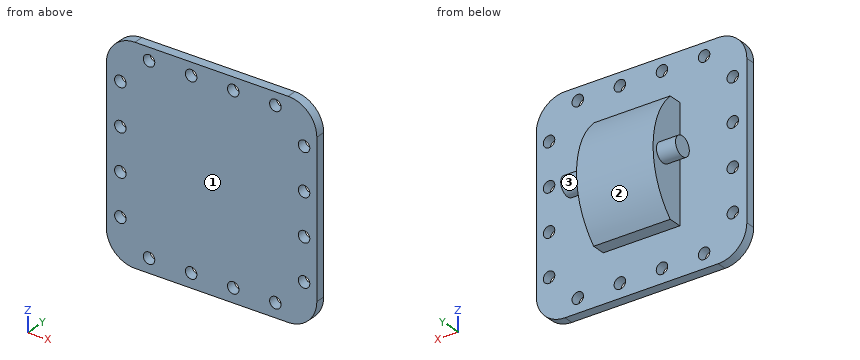
from build123d import *

# Parameters (mm, degrees)
SKETCH1_W                = 110
SKETCH1_H                = 110
BOSS_EXTRUDE1_DEPTH      = 5
FILLET2_R                = 15
FILLET3_R                = 15
FILLET4_R                = 15
FILLET5_R                = 15
SKETCH2_W                = 40
SKETCH2_H                = 60
BOSS_EXTRUDE2_DEPTH      = 24
BOSS_EXTRUDE3_DEPTH      = 10
BOSS_EXTRUDE3_DEPTH_BACK = 50
SKETCH4_R                = 5
FILLET6_R                = 10
FILLET7_R                = 10
SKETCH5_R                = 3
CUT_EXTRUDE1_DEPTH       = 10
CUT_EXTRUDE2_DEPTH       = 60


with BuildPart() as part:
    # Sketch1 → Boss-Extrude1 (new body)
    with BuildSketch(Plane(origin=(0, 0, 0), x_dir=(1, 0, 0), z_dir=(0, 1, 0))):
        Rectangle(SKETCH1_W, SKETCH1_H)
    extrude(amount=BOSS_EXTRUDE1_DEPTH)

    # Fillet2
    fillet2_edges = [part.edges().sort_by_distance(p)[0] for p in [
        (55, 2.5, -55),
    ]]
    fillet(fillet2_edges, radius=FILLET2_R)

    # Fillet3
    fillet3_edges = [part.edges().sort_by_distance(p)[0] for p in [
        (-55, 2.5, -55),
    ]]
    fillet(fillet3_edges, radius=FILLET3_R)

    # Fillet4
    fillet4_edges = [part.edges().sort_by_distance(p)[0] for p in [
        (-55, 2.5, 55),
    ]]
    fillet(fillet4_edges, radius=FILLET4_R)

    # Fillet5
    fillet5_edges = [part.edges().sort_by_distance(p)[0] for p in [
        (55, 2.5, 55),
    ]]
    fillet(fillet5_edges, radius=FILLET5_R)

    # Sketch2 → Boss-Extrude2 (add)
    with BuildSketch(Plane(origin=(0, 5, 0), x_dir=(1, 0, 0), z_dir=(0, 1, 0))):
        Rectangle(SKETCH2_W, SKETCH2_H)
    extrude(amount=BOSS_EXTRUDE2_DEPTH)

    # Sketch4 → Boss-Extrude3 (add, two sides: drawn at the far end of the back side and taken through both)
    with BuildSketch(Plane(origin=(20, 0, 0), x_dir=(0, 0, -1), z_dir=(1, 0, 0)).offset(-BOSS_EXTRUDE3_DEPTH_BACK)):
        with Locations((0, 17)):
            Circle(SKETCH4_R)
    extrude(amount=BOSS_EXTRUDE3_DEPTH + BOSS_EXTRUDE3_DEPTH_BACK)

    # Fillet6
    fillet6_edges = [part.edges().sort_by_distance(p)[0] for p in [
        (0, 29, 30),
    ]]
    fillet(fillet6_edges, radius=FILLET6_R)

    # Fillet7
    fillet7_edges = [part.edges().sort_by_distance(p)[0] for p in [
        (0, 29, -30),
    ]]
    fillet(fillet7_edges, radius=FILLET7_R)

    # Sketch5 → Cut-Extrude1 (cut)
    with BuildSketch(Plane.XZ):
        with Locations(Location((48.334696306, -10.581629618, 0), (0, 0, 270))):
            Circle(SKETCH5_R)
        with Locations(Location((48.334696306, 33.418370382, 0), (0, 0, 270))):
            Circle(SKETCH5_R)
        with Locations(Location((-47.665303694, 11.418370382, 0), (0, 0, 270))):
            Circle(SKETCH5_R)
        with Locations(Location((-47.665303694, -10.581629618, 0), (0, 0, 270))):
            Circle(SKETCH5_R)
        with Locations(Location((-47.665303694, -32.581629618, 0), (0, 0, 270))):
            Circle(SKETCH5_R)
        with Locations(Location((-32.665303694, -47.581629618, 0), (0, 0, 270))):
            Circle(SKETCH5_R)
        with Locations(Location((-10.665303694, -47.581629618, 0), (0, 0, 270))):
            Circle(SKETCH5_R)
        with Locations(Location((11.334696306, -47.581629618, 0), (0, 0, 270))):
            Circle(SKETCH5_R)
        with Locations(Location((33.334696306, -47.581629618, 0), (0, 0, 270))):
            Circle(SKETCH5_R)
        with Locations(Location((48.334696306, -32.581629618, 0), (0, 0, 270))):
            Circle(SKETCH5_R)
        with Locations(Location((48.334696306, 11.418370382, 0), (0, 0, 270))):
            Circle(SKETCH5_R)
        with Locations(Location((33.334696306, 48.418370382, 0), (0, 0, 270))):
            Circle(SKETCH5_R)
        with Locations(Location((11.334696306, 48.418370382, 0), (0, 0, 270))):
            Circle(SKETCH5_R)
        with Locations(Location((-10.665303694, 48.418370382, 0), (0, 0, 270))):
            Circle(SKETCH5_R)
        with Locations(Location((-32.665303694, 48.418370382, 0), (0, 0, 270))):
            Circle(SKETCH5_R)
        with Locations(Location((-47.665303694, 33.418370382, 0), (0, 0, 270))):
            Circle(SKETCH5_R)
    extrude(amount=-CUT_EXTRUDE1_DEPTH, mode=Mode.SUBTRACT)

    # Sketch6 → Cut-Extrude2 (cut)
    with BuildSketch(Plane(origin=(20, 0, 0), x_dir=(0, 0, -1), z_dir=(1, 0, 0))):
        with BuildLine():
            Line((30, 19), (30, 12))
            ThreePointArc((30, 12), (0, 24.426406871), (-30, 12))
            Line((-30, 12), (-30, 19))
            ThreePointArc((-30, 19), (-27.071067812, 26.071067812), (-20, 29))
            Line((-20, 29), (20, 29))
            ThreePointArc((20, 29), (27.071067812, 26.071067812), (30, 19))
        make_face()
    extrude(amount=-CUT_EXTRUDE2_DEPTH, mode=Mode.SUBTRACT)


solid = part.part
Check sheet for the modelled part. Datum: model origin and axes. Units: mm. Face numbers are marked on the shaded views. Round coordinates to 2 decimals unless told otherwise and drop trailing zeros. Loops run counter-clockwise (first coordinate to the right, second up) from the corner with the lowest first, then second, coordinate; pieces in that order, holes last. Notation, with made-up numbers: (60.25, 4) -> (104.25, 4) arc R23 ccw to (104.25, 37) -> close; hole circle Ø1 at (51, 17.5). An arc over 180 degrees is marked (long way). Put each result on its own line as item: value. Start each with the question number.
1. Section check B-B (z = 0). Enter the section's corners in (x, y), plus the area to 3 significant figures.
2. Gauge pin test, flat ends, axial feed: pin 1 (7 mm diameter, centred on x = 11.33, z = -47.58, fed in from +Y); pin 2 (5.5 mm diameter, centred on x = 9, y = 9, fed in from +Z); pin 3 (5.5 mm diameter, centred on x = -10.67, z = 48.42, fed in from -Y); pin 4 (12 mm diameter, centred on y = 11.5, z = 21.5, fed in from -X). Record the tip position at first contact, or that the pin passes through.
3. Section check C-C (y = 19). Enter the section's corners in (x, z), plus the area to 3 significant figures.
4. Section check D-D (z = 18.5). Enter the section's corners in (x, y).
5. Scan lines: probe 1 along X at (y, z) = (4, 12.5); probe 2 along Y at (x, z) = (-39, 18.5); probe 3 along Z at (x, y) = (0.5, 6). Record each from-to range of solid material in increasing order.
6. Section check A-A (x = -27.5). Enter the section's corners in (y, z), plus the area to 3 significant figures.
7. Draft check along Y on the marked faces 1, 2 and 3. Enter one of: +Y half, -Y half, draft (parallel to the pull), parting line (faces both ways), or undercut.
Findings:
1. outline: (-55, 0) -> (55, 0) -> (55, 5) -> (20, 5) -> (20, 12) -> (30, 12) -> (30, 22) -> (20, 22) -> (20, 24.43) -> (-20, 24.43) -> (-20, 22) -> (-30, 22) -> (-30, 12) -> (-20, 12) -> (-20, 5) -> (-55, 5) -> close
1. area: 1,530 mm^2
2. pin 1: stops at y = 5
2. pin 2: stops at z = 30
2. pin 3: passes through
2. pin 4: stops at x = -20
3. outline: (-30, -4.58) -> (-20, -4.58) -> (-20, -20.76) -> (20, -20.76) -> (20, -4.58) -> (30, -4.58) -> (30, 4.58) -> (20, 4.58) -> (20, 20.76) -> (-20, 20.76) -> (-20, 4.58) -> (-30, 4.58) -> close
3. area: 1,840 mm^2
4. outline: (-55, 0) -> (55, 0) -> (55, 5) -> (20, 5) -> (20, 20.18) -> (-20, 20.18) -> (-20, 5) -> (-55, 5) -> close
5. probe 1: x = -55 to -50.46, -44.87 to 45.54, 51.13 to 55
5. probe 2: y = 0 to 5
5. probe 3: z = -30 to 30
6. outline: (0, -55) -> (5, -55) -> (5, 55) -> (0, 55) -> close; circle Ø10 at (17, 0)
6. area: 629 mm^2
7. face 1: -Y half
7. face 2: +Y half
7. face 3: undercut
